For this review, use the dimensioned drawing (mm, ordinates from the lowest corner) and the shaded views. A direction names the side the tool comes from. Give positions to 0.01 mm unless a question says otherwise; leave off trailing zeros. Loops run counter-clockwise (first coordinate to the right, second up) from the corner with the lowest first, then second, coordinate; pieces in that order, holes last. Notation, with made-up numbers: (30, -22.5) -> (83, -22.5) arc R19 cw to (83, 13.5) -> close; hole circle Ø7 at (-28, 53.25). An arc over 180 degrees is marked (long way). Use a Markdown table: item, result. Add a question column.
1. Add section A-A (y = 6.5). State the section outline as (x, z) points.
2. Add section D-D (x = 3.5). State the section outline as (y, z) points.
3. Add section C-C (z = 8.75). State the section outline as (x, y) points, and give its area (3 significant figures).
4. To check wall thickness, follow line 1 (Z direction, x = 1.5, y = 3); line 2 (Y direction, x = 6.5, z = 6.5); line 3 (Y direction, x = 6.5, z = 13.75). State the ranges of each line that lie inside material, in increasing order.
5. For the marked faces 4 and 5, list the 3-axis set-ups (+Z, -Z, +X, -X, +Y, -Y) from which the entire face can be reached by the end or side of a thin tool; tool diameter is ignored.
6. For pin 1 Ø1.5 at (x, z) = (9.5, 9) entering from +Y; pin 2 Ø1 at (x, z) = (3.5, 17.5) entering from -Y; pin 3 Ø1.8 at (x, y) = (6.5, 6.5) entering from +Z; pin 4 Ø5 at (x, z) = (2, 14) entering from +Y, all flat-tipped, find the tip position at first contact; note any pin that passes through.
7. Draft analysis for pull direction X (two halves, no side actions). For the marked faces 1, 2 and 3, state which applies: pulls with the +X half, pulls with the -X half, needs draft (parallel to the pull), parting line crosses it, or undercut.
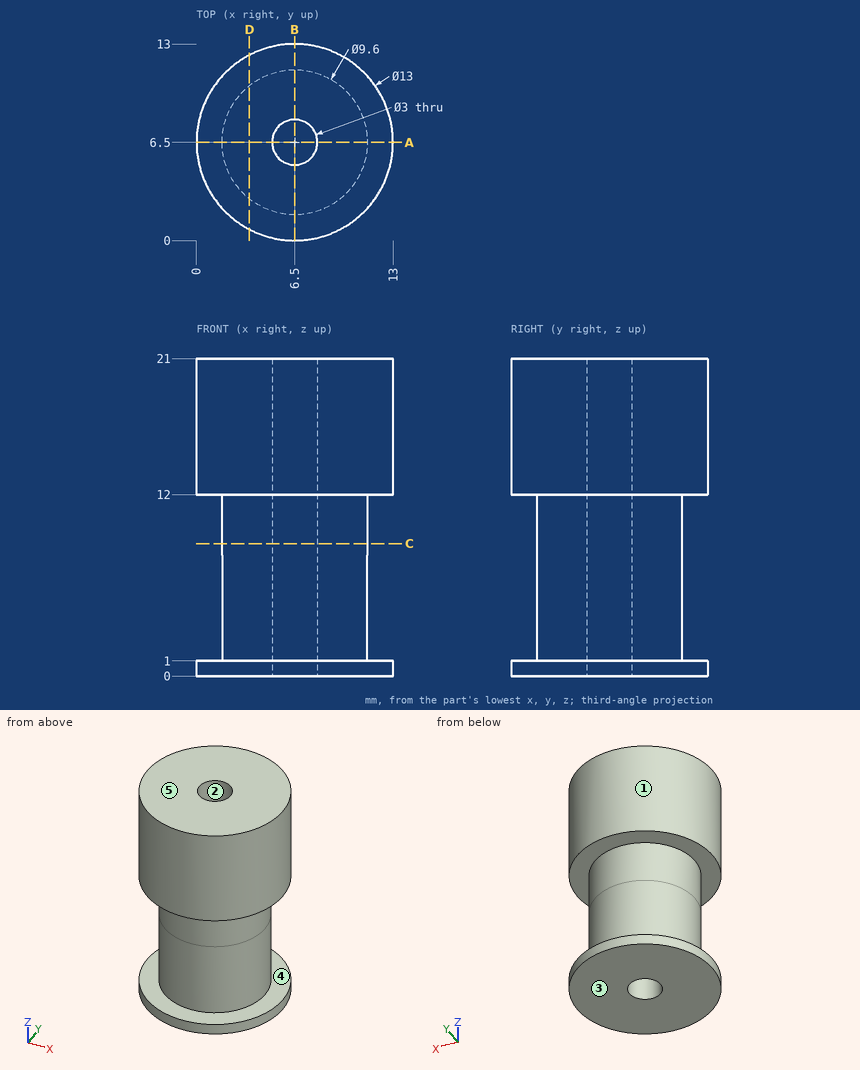
Taken from the geometry:
| question | item | result |
|---|---|---|
| 1 | outline | (0, 0) -> (5, 0) -> (5, 21) -> (0, 21) -> (0, 12) -> (1.7, 12) -> (1.7, 1) -> (0, 1) -> close; (8, 0) -> (13, 0) -> (13, 1) -> (11.3, 1) -> (11.3, 12) -> (13, 12) -> (13, 21) -> (8, 21) -> close |
| 2 | outline | (0.73, 0) -> (12.27, 0) -> (12.27, 1) -> (10.25, 1) -> (10.25, 12) -> (12.27, 12) -> (12.27, 21) -> (0.73, 21) -> (0.73, 12) -> (2.75, 12) -> (2.75, 1) -> (0.73, 1) -> close |
| 3 | outline | circle Ø9.6 at (6.5, 6.5); hole circle Ø3 at (6.5, 6.5) |
| 3 | area | 65.3 mm^2 |
| 4 | line 1 | z = 0 to 1, 12 to 21 |
| 4 | line 2 | y = 1.7 to 5, 8 to 11.3 |
| 4 | line 3 | y = 0 to 5, 8 to 13 |
| 5 | face 4 | none |
| 5 | face 5 | +Z, +X, -X, +Y, -Y |
| 6 | pin 1 | stops at y = 10.74 |
| 6 | pin 2 | stops at y = 0.5 |
| 6 | pin 3 | passes through |
| 6 | pin 4 | stops at y = 12.68 |
| 7 | face 1 | parting line crosses it |
| 7 | face 2 | undercut |
| 7 | face 3 | needs draft |
